```python
from build123d import *

# Parameters (mm, degrees)
SKETCH1_W               = 203.2
SKETCH1_H               = 101.6
BOSS_EXTRUDE1_DEPTH     = 6.35
SKETCH2_R               = 9.525
CUT_EXTRUDE1_DEPTH      = 228.273233136
SKETCH3_R               = 6.35
CUT_EXTRUDE2_DEPTH      = 228.273233136
MIRROR2_COPY_1_SKETCH_R = 6.35
MIRROR2_COPY_1_DEPTH    = 228.273233136
SKETCH4_R               = 3.175
CUT_EXTRUDE3_DEPTH      = 228.273233136
CIRPATTERN1_COUNT       = 4


with BuildPart() as part:
    # Sketch1 → Boss-Extrude1 (new body)
    with BuildSketch(Plane(origin=(0, 0, 0), x_dir=(1, 0, 0), z_dir=(0, 1, 0))):
        with Locations((101.6, 50.8)):
            Rectangle(SKETCH1_W, SKETCH1_H)
    extrude(amount=BOSS_EXTRUDE1_DEPTH)

    # Sketch2 → Cut-Extrude1 (cut, through all)
    with BuildSketch(Plane(origin=(0, 6.35, 0), x_dir=(1, 0, 0), z_dir=(0, 1, 0))):
        with Locations(Location((63.5, 50.8, 0), (0, 0, 270))):
            Circle(SKETCH2_R)
    extrude(amount=-CUT_EXTRUDE1_DEPTH, mode=Mode.SUBTRACT)

    # Sketch3 → Cut-Extrude2 (cut, through all)
    with BuildSketch(Plane(origin=(0, 6.35, 0), x_dir=(1, 0, 0), z_dir=(0, 1, 0))):
        with Locations(Location((12.7, 88.9, 0), (0, 0, 270))):
            Circle(SKETCH3_R)
    cut_extrude2 = extrude(amount=-CUT_EXTRUDE2_DEPTH, mode=Mode.SUBTRACT)

    # Mirror1: Cut-Extrude2 across plane
    add(cut_extrude2.mirror(Plane.XY.offset(-50.8)), mode=Mode.SUBTRACT)

    # Mirror2: Cut-Extrude2 across plane
    add(cut_extrude2.mirror(Plane.ZY.offset(-101.6)), mode=Mode.SUBTRACT)

    # Mirror2 copy 1 sketch → Mirror2 copy 1 (cut, through all)
    with BuildSketch(Plane(origin=(203.2, 6.35, -101.6), x_dir=(-1, 0, 0), z_dir=(0, 1, 0))):
        with Locations(Location((12.7, 88.9, 0), (0, 0, 270))):
            Circle(MIRROR2_COPY_1_SKETCH_R)
    extrude(amount=-MIRROR2_COPY_1_DEPTH, mode=Mode.SUBTRACT)

    # Sketch4 → Cut-Extrude3 (cut, through all)
    with BuildSketch(Plane(origin=(0, 6.35, 0), x_dir=(1, 0, 0), z_dir=(0, 1, 0))):
        with Locations(Location((36.693935479, 77.606064521, 0), (0, 0, 270))):
            Circle(SKETCH4_R)
    cut_extrude3 = extrude(amount=-CUT_EXTRUDE3_DEPTH, mode=Mode.SUBTRACT)

    # CirPattern1: Cut-Extrude3 ×4 about axis
    cirpattern1_axis = Axis((63.5, 0, -50.8), (0, 1, 0))
    for i in range(1, CIRPATTERN1_COUNT):
        add(cut_extrude3.rotate(cirpattern1_axis, i * 360 / CIRPATTERN1_COUNT), mode=Mode.SUBTRACT)


solid = part.part
```
Verification items for the finished model (mm, model axes). Give positions to 0.01 mm unless a question says otherwise; leave off trailing zeros. Order: outer loops, then holes, each group sorted by start corner. A loop starts at its lowest first (then second) coordinate and runs counter-clockwise, first axis right, second up. Notation, with made-up numbers: (26.25, -37.75) -> (81.25, -37.75) arc R30 cw to (81.25, -1.75) -> close; hole circle Ø8 at (5.25, 41). An arc over 180 degrees is marked (long way). Use a Markdown table: item, result.
1) Section check D-D, the plane x = 12.7. Record the boundary of the cut face in (y, z).
Results:
| item | result |
|---|---|
| outline | (0, -101.6) -> (6.35, -101.6) -> (6.35, -95.25) -> (0, -95.25) -> close; (0, -82.55) -> (6.35, -82.55) -> (6.35, -19.05) -> (0, -19.05) -> close; (0, -6.35) -> (6.35, -6.35) -> (6.35, 0) -> (0, 0) -> close |
2) Section check B-B, the plane z = -50.8. Record the boundary of the cut face in (x, y) (3 decimals).
Results:
| item | result |
|---|---|
| outline | (0, 0) -> (53.975, 0) -> (53.975, 6.35) -> (0, 6.35) -> close; (73.025, 0) -> (203.2, 0) -> (203.2, 6.35) -> (73.025, 6.35) -> close |
3) Material ranges on probe 1 along X at (y, z) = (4.5, -12.7); probe 2 along X at (y, z) = (3, -24.5); probe 3 along Z at (x, y) = (190.5, 5.25), recorded low to high.
Results:
| item | result |
|---|---|
| probe 1 | 0 to 6.35, 19.05 to 184.15, 196.85 to 203.2 |
| probe 2 | 0 to 33.56, 39.83 to 87.17, 93.44 to 203.2 |
| probe 3 | -101.6 to -95.25, -82.55 to -19.05, -6.35 to 0 |
4) Mould release check, pull along X, two halves, no side actions. Record for faces 1 (the flat face through (100, 3, 0)), 2 (the cylindrical face through (184.2, 3.2, -11.9)), 3 (the flat face through (203.2, 3, -50)): pulls with the +X half, pulls with the -X half, needs draft (parallel to the pull), parting line crosses it, or undercut.
Results:
| item | result |
|---|---|
| face 1 | needs draft |
| face 2 | undercut |
| face 3 | pulls with the +X half |
5) Section check C-C, the plane x = 63.5. Record the boundary of the cut face in (y, z) (3 decimals), then the cut area to 3 significant figures.
Results:
| item | result |
|---|---|
| outline | (0, -101.6) -> (6.35, -101.6) -> (6.35, -60.325) -> (0, -60.325) -> close; (0, -41.275) -> (6.35, -41.275) -> (6.35, 0) -> (0, 0) -> close |
| area | 524 mm² |
6) Section check A-A, the plane z = -88.9. Record the boundary of the cut face in (x, y).
Results:
| item | result |
|---|---|
| outline | (0, 0) -> (6.35, 0) -> (6.35, 6.35) -> (0, 6.35) -> close; (19.05, 0) -> (184.15, 0) -> (184.15, 6.35) -> (19.05, 6.35) -> close; (196.85, 0) -> (203.2, 0) -> (203.2, 6.35) -> (196.85, 6.35) -> close |
